Geometry: final body of the model. Coordinates: model frame, mm. Face numbers are marked on the shaded views. A direction names the side the tool comes from. Give positions to 0.01 mm unless a question says otherwise; leave off trailing zeros. Loops run counter-clockwise (first coordinate to the right, second up) from the corner with the lowest first, then second, coordinate; pieces in that order, holes last. Notation, with made-up numbers: (39.25, 88) -> (55.25, 88) arc R14 ccw to (55.25, 106) -> close; hole circle Ø2 at (35.5, 46). An arc over 180 degrees is marked (long way). Answer in a Markdown table with one row per item. Add a question column.
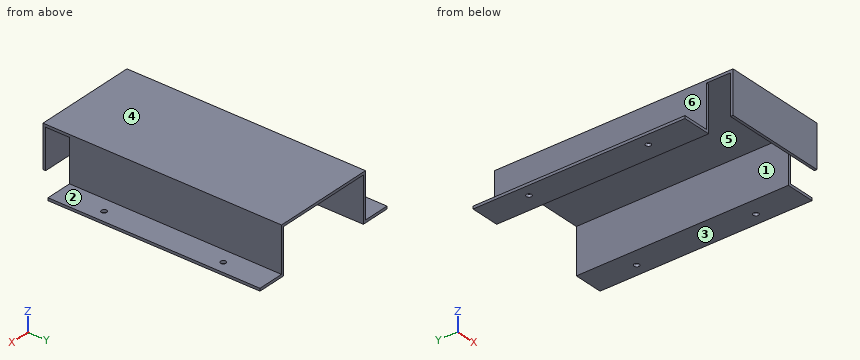
from build123d import *

# Parameters (mm, degrees)
F0_W      = 39
F0_H      = 90
F1_DEPTH  = 1
F2_W      = 1
F2_H      = 90
F3_DEPTH  = 17
F4_W      = 90
F4_H      = 1
F5_DEPTH  = 10
F6_W      = 10
F6_H      = 18
F7_DEPTH  = 11
F8_W      = 38
F8_H      = 1
F9_DEPTH  = 15
F10_R     = 1
F11_DEPTH = 1


with BuildPart() as f1:
    # F0 (on Top) → F1 (new body)
    with BuildSketch(Plane.XY):
        Rectangle(F0_W, F0_H)
    extrude(amount=F1_DEPTH)

    # F2 (on face) → F3 (join)
    with BuildSketch(Plane(origin=(0, 0, 0), x_dir=(1, 0, 0), z_dir=(0, 0, -1))):
        with Locations((19, 0)):
            Rectangle(F2_W, F2_H)
    extrude(amount=F3_DEPTH)

    # F4 (on face) → F5 (join)
    with BuildSketch(Plane.YZ.offset(19.5)):
        with Locations((0, -16.5)):
            Rectangle(F4_W, F4_H)
    extrude(amount=F5_DEPTH)

    # F6 (on face) → F7 (cut, through all)
    with BuildSketch(Plane.YZ.offset(29.5)):
        with Locations((-40, -8)):
            Rectangle(F6_W, F6_H)
    extrude(amount=-F7_DEPTH, mode=Mode.SUBTRACT)

    # F8 (on face) → F9 (join)
    with BuildSketch(Plane(origin=(0, 0, 0), x_dir=(1, 0, 0), z_dir=(0, 0, -1))):
        with Locations((-0.5, 44.5)):
            Rectangle(F8_W, F8_H)
    extrude(amount=F9_DEPTH)

    # F10 (on face) → F11 (cut, through all)
    with BuildSketch(Plane.XY.offset(-16)):
        with Locations((25, 27.5)):
            Circle(F10_R)
        with Locations((25, -17.5)):
            Circle(F10_R)
    extrude(amount=-F11_DEPTH, mode=Mode.SUBTRACT)

    # F12: F1 across plane


with BuildPart() as f1_1:
    add(f1.part)
    add(f1.part.mirror(Plane.YZ))


solid = f1_1.part
(1) Reachability of the marked faces 1, 2 and 3 from +Z, -Z, +X, -X, +Y, -Y: full face, straight path, thin tool, end or side. Return the list, or none.
(2) Cut plane A-A on z = -5.75. Return the cut outline in (x, y).
(3) Cut plane C-C on y = 27.5. Return the cut outline in (x, z).
(4) Cut plane D-D on y = 13. Return the cut outline in (x, z).
(5) Draft query along X for the marked faces 4, 5 and 6. Return one class per face: +X half, -X half, draft (parallel to the pull), parting line (faces both ways), or undercut.
(6) Cut plane B-B on x = 25. Return the cut outline in (y, z), then the cut area to 3 significant figures.
(7) Pin query (flat end, axial travel): pin 1 Ø5 at (y, z) = (-5, -4) entering from +X; pin 2 Ø11.5 at (x, y) = (-4.5, 18) entering from -Z; pin 3 Ø5.5 at (x, z) = (23.5, -6) entering from -Y; pin 4 Ø2 at (x, z) = (-3.5, -13) entering from +Y. Return the tip coordinate at first contact, or that it passes through.
(8) Material intervals for line 1 along Y through (x, z) = (-25, -16.3); line 2 along X through (y, z) = (-1, -10.5); line 3 along Y through (x, z) = (16, -10.75), sorted ascending. Write a range as from..to.
Answer list:
| question | item | result |
|---|---|---|
| 1 | face 1 | -Z, +Y |
| 1 | face 2 | +Z, +X, +Y, -Y |
| 1 | face 3 | -Z, +X, -X, +Y, -Y |
| 2 | outline | (-19.5, -45) -> (19.5, -45) -> (19.5, -44) -> (-19.5, -44) -> close; (-19.5, -35) -> (-18.5, -35) -> (-18.5, 45) -> (-19.5, 45) -> close; (18.5, -35) -> (19.5, -35) -> (19.5, 45) -> (18.5, 45) -> close |
| 3 | outline | (-29.5, -17) -> (-26, -17) -> (-26, -16) -> (-29.5, -16) -> close; (-24, -17) -> (-18.5, -17) -> (-18.5, 0) -> (18.5, 0) -> (18.5, -17) -> (24, -17) -> (24, -16) -> (19.5, -16) -> (19.5, 1) -> (-19.5, 1) -> (-19.5, -16) -> (-24, -16) -> close; (26, -17) -> (29.5, -17) -> (29.5, -16) -> (26, -16) -> close |
| 4 | outline | (-29.5, -17) -> (-18.5, -17) -> (-18.5, 0) -> (18.5, 0) -> (18.5, -17) -> (29.5, -17) -> (29.5, -16) -> (19.5, -16) -> (19.5, 1) -> (-19.5, 1) -> (-19.5, -16) -> (-29.5, -16) -> close |
| 5 | face 4 | draft |
| 5 | face 5 | undercut |
| 5 | face 6 | -X half |
| 6 | outline | (-35, -17) -> (-18.5, -17) -> (-18.5, -16) -> (-35, -16) -> close; (-16.5, -17) -> (26.5, -17) -> (26.5, -16) -> (-16.5, -16) -> close; (28.5, -17) -> (45, -17) -> (45, -16) -> (28.5, -16) -> close |
| 6 | area | 76.0 mm² |
| 7 | pin 1 | stops at x = 19.5 |
| 7 | pin 2 | stops at z = 0 |
| 7 | pin 3 | passes through |
| 7 | pin 4 | stops at y = -44 |
| 8 | line 1 | y = -35..-18.5, -16.5..26.5, 28.5..45 |
| 8 | line 2 | x = -19.5..-18.5, 18.5..19.5 |
| 8 | line 3 | y = -45..-44 |
